```python
from build123d import *

# Parameters (mm, degrees)
SKETCH_1_R      = 1.6
EXTRUDE_1_DEPTH = 3


with BuildPart() as part:
    # 草图1 → 凸台-拉伸1 (new body)
    with BuildSketch(Plane.XY):
        with BuildLine():
            Line((3, 0), (145, 0))
            ThreePointArc((145, 0), (147.121320344, 0.878679656), (148, 3))
            Line((148, 3), (148, 68))
            ThreePointArc((148, 68), (147.121320344, 70.121320344), (145, 71))
            Line((145, 71), (3, 71))
            ThreePointArc((3, 71), (0.878679656, 70.121320344), (0, 68))
            Line((0, 68), (0, 3))
            ThreePointArc((0, 3), (0.878679656, 0.878679656), (3, 0))
        make_face()
        with Locations((3, 3)):
            Circle(SKETCH_1_R, mode=Mode.SUBTRACT)
        with Locations((145, 3)):
            Circle(SKETCH_1_R, mode=Mode.SUBTRACT)
        with Locations((145, 68)):
            Circle(SKETCH_1_R, mode=Mode.SUBTRACT)
        with Locations((3, 68)):
            Circle(SKETCH_1_R, mode=Mode.SUBTRACT)
        with Locations((14, 63)):
            Circle(SKETCH_1_R, mode=Mode.SUBTRACT)
        with Locations((63, 63)):
            Circle(SKETCH_1_R, mode=Mode.SUBTRACT)
        with Locations((63, 5)):
            Circle(SKETCH_1_R, mode=Mode.SUBTRACT)
        with Locations((14, 5)):
            Circle(SKETCH_1_R, mode=Mode.SUBTRACT)
        with Locations(Location((85, 63, 0), (0, 0, 180))):
            Circle(SKETCH_1_R, mode=Mode.SUBTRACT)
        with Locations(Location((85, 5, 0), (0, 0, 180))):
            Circle(SKETCH_1_R, mode=Mode.SUBTRACT)
        with Locations(Location((134, 5, 0), (0, 0, 180))):
            Circle(SKETCH_1_R, mode=Mode.SUBTRACT)
        with Locations(Location((134, 63, 0), (0, 0, 180))):
            Circle(SKETCH_1_R, mode=Mode.SUBTRACT)
    extrude(amount=EXTRUDE_1_DEPTH)


solid = part.part
```
Check sheet for the modelled part. Datum: model origin and axes. Units: mm. Give positions to 0.01 mm unless a question says otherwise; leave off trailing zeros. Write each loop counter-clockwise with the first axis right and the second up, starting at its lowest first coordinate (ties: lowest second). Pieces come first, ordered by that corner, then holes. Notation, with made-up numbers: (-0.5, 24.25) - (42.5, 24.25) arc R15 cw to (42.5, 48.25) - close; hole circle Ø2 at (37, 77.25). An arc over 180 degrees is marked (long way). Answer as a JSON object with one key per item and string values. Group by question number.
1) Thickness scan on probe 1 along Y at (x, z) = (3, 2.25); probe 2 along Y at (x, z) = (62.5, 0.45); probe 3 along X at (y, z) = (6, 2.35). Record the ranges inside material, lowest first. Write a range as from..to.
2) Release check for a two-part mould opening along Y. For faces 1 (the face through (147.14, 70.1, 1.48)), 2 (the face through (13.792, 64.586, 1.479)), 3 (the face through (0.86, 0.9, 1.48)) record: pulls with the +Y half, pulls with the -Y half, needs draft (parallel to the pull), parting line crosses it, or undercut.
3) Sectioned sample at B-B (y = 63). Record the cut outline in (x, z), then the cut area to 3 significant figures.
4) Sectioned sample at A-A (x = 14). Record the cut outline in (y, z).
5) Depth check by flat-ended pin: P1, Ø1.9, axis at x = 85, y = 63, coming from the +Z side. Enter the tip coordinate at first touch or a pass-through.
Geometry results:
{
 "1": {"probe 1": "y = 0..1.4, 4.6..66.4, 69.6..71", "probe 2": "y = 0..3.48, 6.52..61.48, 64.52..71", "probe 3": "x = 0..12.75, 15.25..61.75, 64.25..83.75, 86.25..132.75, 135.25..148"},
 "2": {"face 1": "pulls with the +Y half", "face 2": "undercut", "face 3": "pulls with the -Y half"},
 "3": {"outline": "(0, 0) - (12.4, 0) - (12.4, 3) - (0, 3) - close; (15.6, 0) - (61.4, 0) - (61.4, 3) - (15.6, 3) - close; (64.6, 0) - (83.4, 0) - (83.4, 3) - (64.6, 3) - close; (86.6, 0) - (132.4, 0) - (132.4, 3) - (86.6, 3) - close; (135.6, 0) - (148, 0) - (148, 3) - (135.6, 3) - close", "area": "406 mm^2"},
 "4": {"outline": "(0, 0) - (3.4, 0) - (3.4, 3) - (0, 3) - close; (6.6, 0) - (61.4, 0) - (61.4, 3) - (6.6, 3) - close; (64.6, 0) - (71, 0) - (71, 3) - (64.6, 3) - close"},
 "5": {"P1": "passes through"}
}
